Design review of the part shown in the three views and the two pictorial views. Dimensions are in mm from the part's minimum x, y and z. Round coordinates to 2 decimals unless told otherwise and drop trailing zeros. Order: outer loops, then holes, each group sorted by start corner. A loop starts at its lowest first (then second) coordinate and runs counter-clockwise, first axis right, second up.
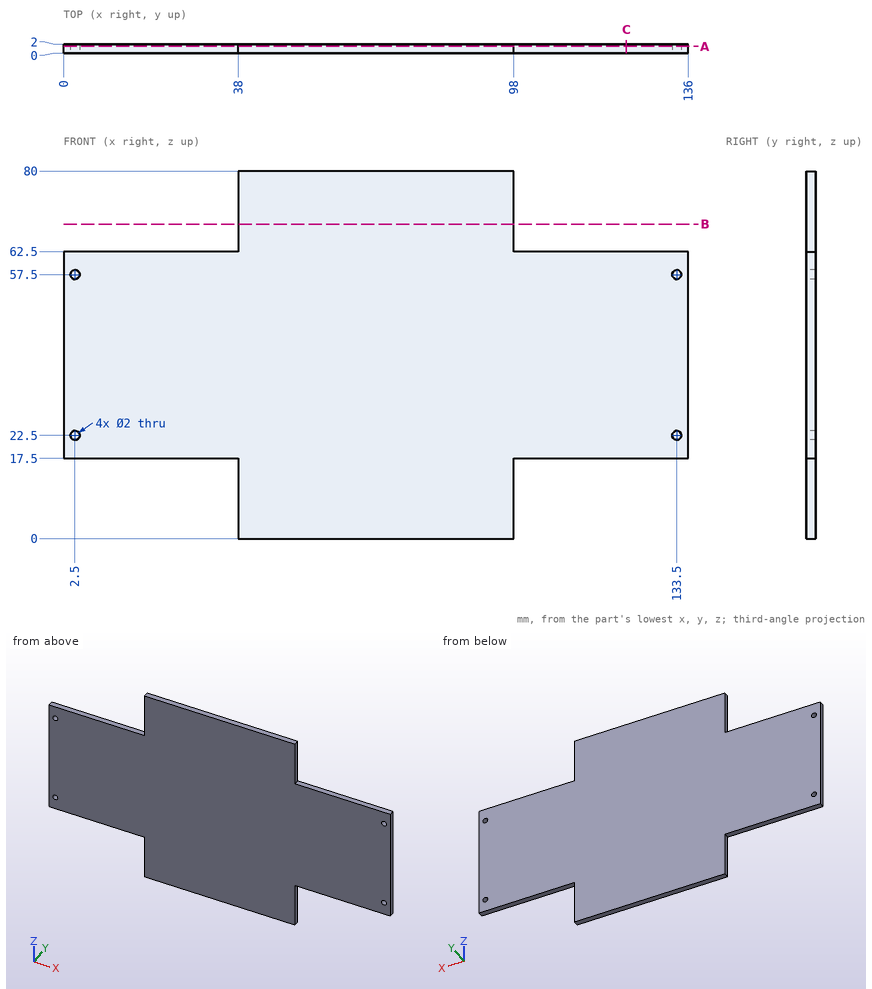
(1) Wall thickness on L1, parallel to X at y = 0.95, z = 57.5; L2, parallel to Z at x = 2.5, y = 1.1; L3, parallel to X at y = 1.85, z = 11.5: over which ranges is each line inside the solid? List them lowest first.
(2) Add section C-C on x = 122.5. Give the boundary of the cut face in (y, z).
(3) Clearance check with flat-ended pins moving along their axes: P1, Ø1.6, axis at x = 133.5, z = 57.5, coming from the +Y side; P2, Ø1, axis at y = 0.5, z = 71, coming from the +X side; P3, Ø2.5, axis at x = 2.5, z = 57.5, coming from the +Y side; P4, Ø0.6, axis at x = 17, y = 0.5, coming from the -Z side. State where each tip first meets the part, or that it passes through.
(4) Add section A-A on y = 1.5. Give the boundary of the cut face in (x, z), plus the area to 3 significant figures.
(5) Add section B-B on z = 68.5. Give the boundary of the cut face in (x, y), plus the area to 3 significant figures.
Here are the results:
1. L1: x = 0 to 1.5, 3.5 to 132.5, 134.5 to 136
1. L2: z = 17.5 to 21.5, 23.5 to 56.5, 58.5 to 62.5
1. L3: x = 38 to 98
2. outline: (0, 17.5) - (2, 17.5) - (2, 62.5) - (0, 62.5) - close
3. P1: passes through
3. P2: stops at x = 98
3. P3: stops at y = 2
3. P4: stops at z = 17.5
4. outline: (0, 17.5) - (38, 17.5) - (38, 0) - (98, 0) - (98, 17.5) - (136, 17.5) - (136, 62.5) - (98, 62.5) - (98, 80) - (38, 80) - (38, 62.5) - (0, 62.5) - close; hole circle Ø2 at (2.5, 22.5); hole circle Ø2 at (2.5, 57.5); hole circle Ø2 at (133.5, 22.5); hole circle Ø2 at (133.5, 57.5)
4. area: 8,210 mm2
5. outline: (38, 0) - (98, 0) - (98, 2) - (38, 2) - close
5. area: 120 mm2
